Answer from the drawing. Dimensions are ordinates in mm from the lowest x, y and z of the part. A direction names the side the tool comes from. Round coordinates to 2 decimals unless told otherwise and drop trailing zeros. Write each loop counter-clockwise with the first axis right and the second up, starting at its lowest first coordinate (ties: lowest second). Pieces come first, ordered by that corner, then holes. Notation, with made-up numbers: (49.25, 24) -> (67.25, 24) arc R18 cw to (67.25, 49) -> close; hole circle Ø8 at (1.5, 6). An arc over 180 degrees is marked (long way). Answer as a JSON object with one key per item and string values. Group by question number.
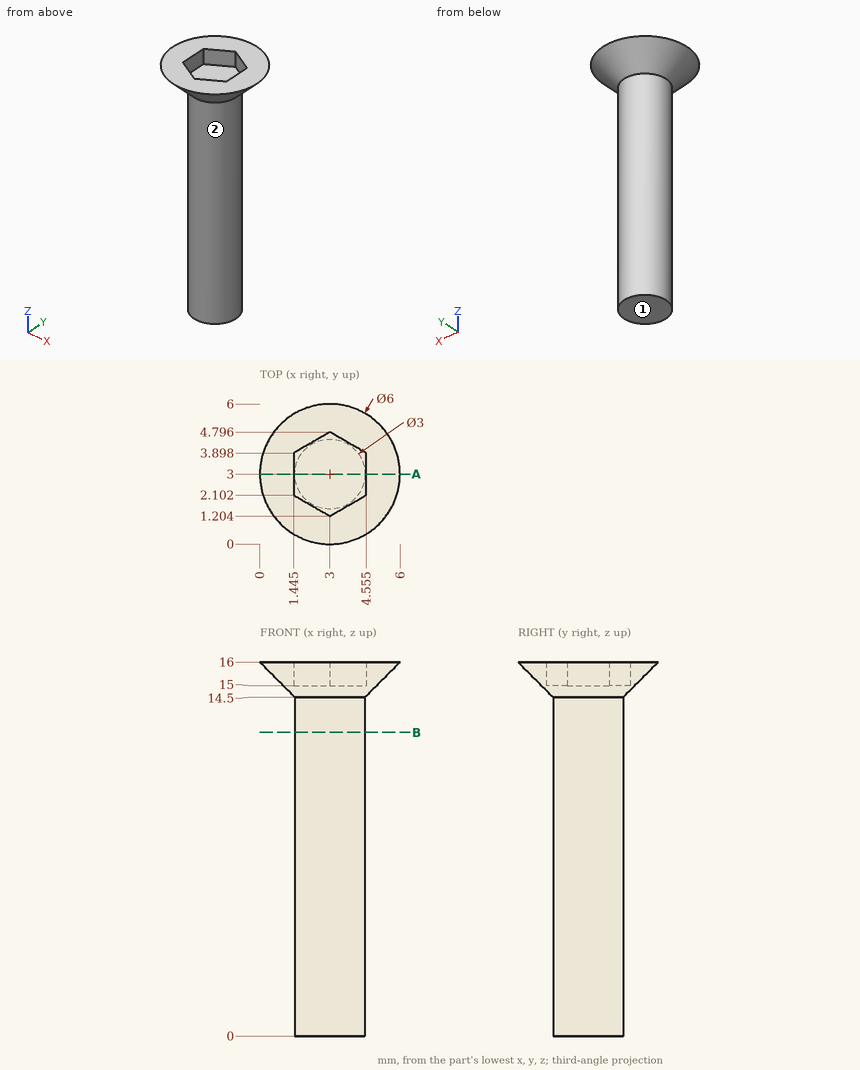
1) Straight lines are drawn through the part: L1, parallel to Z at x = 2.55, y = 3.3; L2, parallel to X at y = 2.9, z = 9.25. For each, find the intervals that lie inside material, in ascending order.
2) A tool of negligible diameter and unlimited length cuts with its end or side. For the marked faces 1 and 2, from which of +Z, -Z, +X, -X, +Y, -Y can it reach the whole face along a straight path? Write none if from no direction.
3) A cutting plane is placed at B-B on z = 13. Determine the outline of the cut face in (x, y).
4) A cutting plane is placed at A-A on y = 3. Determine the outline of the cut face in (x, z) (1 decimal).
5) Each of these flat-tipped pins is pushed along its axis until it touches: P1, Ø1.5, axis at x = 1.5, y = 3.5, coming from the -Z side; P2, Ø0.5, axis at y = 2.5, z = 15.5, coming from the -X side; P3, Ø0.5, axis at y = 3, z = 15.5, coming from the +X side; P4, Ø0.9, axis at x = 3, y = 2.5, coming from the +Z side. Where does it stop, or does it pass through?
Established:
{
 "1": {"L1": "z = 0 to 15", "L2": "x = 1.5 to 4.5"},
 "2": {"face 1": "-Z, +X, -X, +Y, -Y", "face 2": "-Z"},
 "3": {"outline": "circle Ø3 at (3, 3)"},
 "4": {"outline": "(0, 16) -> (1.5, 14.5) -> (1.5, 0) -> (4.5, 0) -> (4.5, 14.5) -> (6, 16) -> (4.6, 16) -> (4.6, 15) -> (1.4, 15) -> (1.4, 16) -> close"},
 "5": {"P1": "stops at z = 0", "P2": "stops at x = 0.29", "P3": "stops at x = 5.75", "P4": "stops at z = 15"}
}
